from build123d import *

# Parameters (mm, degrees)
SKETCH2_W          = 1
SKETCH2_H          = 6.5
CUT_EXTRUDE1_DEPTH = 1.5


with BuildPart() as part:
    # Sketch1 → Revolve1 (revolve)
    with BuildSketch(Plane.XY):
        Polygon((0, 0), (-23, 0), (-23, 2), (-3, 2), (-3, 3.25), (0, 3.25), align=None)
    revolve(axis=Axis((0, 0, 0), (-1, 0, 0)))

    # Sketch2 → Cut-Extrude1 (cut)
    with BuildSketch(Plane(origin=(0, 0, 0), x_dir=(0, 0, -1), z_dir=(1, 0, 0))):
        Rectangle(SKETCH2_W, SKETCH2_H)
    extrude(amount=-CUT_EXTRUDE1_DEPTH, mode=Mode.SUBTRACT)


solid = part.part
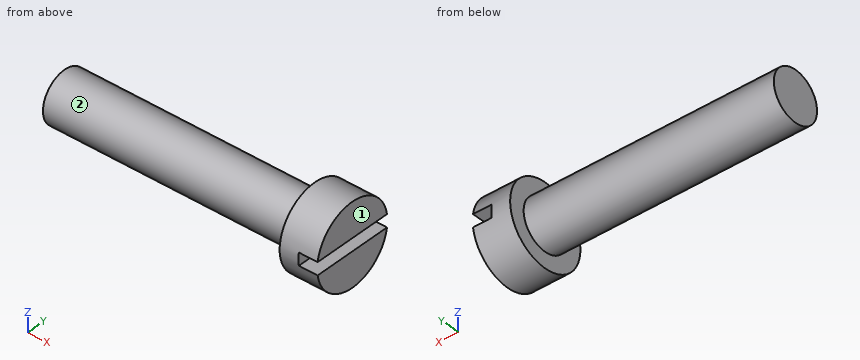
Can you work these out from the model? Positions are in its coordinate system, mm. Face numbers are marked on the shaded views. A direction names the side the tool comes from. Coordinates: 2 decimals unless noted, no trailing zeros. Order: outer loops, then holes, each group sorted by start corner. A loop starts at its lowest first (then second) coordinate and runs counter-clockwise, first axis right, second up. Notation, with made-up numbers: M 44.25,36.25 L 85.25,36.25 A20 ccw 85.25,58.25 Z; hole C 59,39.25 d2. An arc over 180 degrees is marked long. Write item = value, one per line.
(1) Suppose I cut it at A-A on y = 0. Please give me the cut outline in (x, z), plus the area to 3 significant figures.
Results are:
outline = M -23,-2 L -3,-2 L -3,-3.25 L 0,-3.25 L 0,-0.5 L -1.5,-0.5 L -1.5,0.5 L 0,0.5 L 0,3.25 L -3,3.25 L -3,2 L -23,2 Z
area = 98.0 mm2
(2) Suppose I cut it at B-B on z = 0. Please give me the cut outline in (x, y), plus the area to 4 significant figures.
Results are:
outline = M -23,-2 L -3,-2 L -3,-3.25 L -1.5,-3.25 L -1.5,3.25 L -3,3.25 L -3,2 L -23,2 Z
area = 89.75 mm2
(3) For pin 1 Ø0.5 at (y, z) = (-1.5, 0) entering from +X; pin 2 Ø2 at (x, y) = (-16, -1) entering from +Z; pin 3 Ø1.5 at (x, z) = (-6.5, 0) entering from +Y, each with a flat end and sliding along its axis, tell me the tip position at first contact or that it passes through.
Results are:
pin_1 = -1.5
pin_2 = 2
pin_3 = 2
(4) For the marked faces 1 and 2, which set-ups out of +Z, -Z, +X, -X, +Y, -Y let a thin tool reach every point of the face, with its end or its side?
Results are:
face_1 = +Z, -Z, +X, +Y, -Y
face_2 = -X
(5) I need wall thicknesses on line 1 along X through (y, z) = (-2.5, -2); line 2 along Z through (x, y) = (-17, 0); line 3 along Z through (x, y) = (-20, -0.75). Which ranges of each line are inside material? Lowest first, please. Write a range as [from, to].
Results are:
line_1 = [-3, 0]
line_2 = [-2, 2]
line_3 = [-1.85, 1.85]
(6) Suppose I cut it at C-C on x = -10. Please give me the cut outline in (y, z), plus the area to 3 significant figures.
Results are:
outline = C 0,0 d4
area = 12.6 mm2
(7) Suppose I cut it at D-D on y = -1.25. Please give me the cut outline in (x, z), plus the area to 4 significant figures.
Results are:
outline = M -23,-1.56 L -3,-1.56 L -3,-3 L 0,-3 L 0,-0.5 L -1.5,-0.5 L -1.5,0.5 L 0,0.5 L 0,3 L -3,3 L -3,1.56 L -23,1.56 Z
area = 78.95 mm2
